Autodesk Fusion 360 part; units mm, degrees
sketch "Sketch1" plane through (0, 0, 0) normal (0, 0, 1) x (1, 0, 0)
  line L0 (4, 2) -> (-4, 2)
  line L1 (-4, 2) -> (-4, -2)
  line L2 (-4, -2) -> (4, -2)
  line L3 (4, -2) -> (4, 2)
  line L4 (4, 2) -> (-4, -2) construction
  line L5 (-4, 2) -> (4, -2) construction
  line L6 (-4, -2) -> (-17, -2)
  line L7 (-17, -2) -> (-17, 10)
  line L8 (-17, 10) -> (0, 10)
  line L9 (-4, 0) -> (-15, 0)
  line L10 (-15, 0) -> (-15, 8)
  line L11 (-15, 8) -> (0, 8)
  line L12 (0, 1.75) -> (0, 22.5)
  line L13 (15, 8) -> (0, 8)
  line L14 (17, 10) -> (0, 10)
  line L15 (17, -2) -> (17, 10)
  line L16 (15, 0) -> (15, 8)
  line L17 (4, 0) -> (15, 0)
  line L18 (4, -2) -> (17, -2)
  line L19 (-17, 10) -> (-23, 10)
  line L20 (-23, 10) -> (-23, 4)
  line L21 (-17, -2) -> (-17, 10)
  circle A0 centre (-20, 7) radius 1.75
  line L22 (-23, 4) -> (-17, -2)
  line L23 (17, 10) -> (23, 10)
  line L24 (23, 10) -> (23, 4)
  line L25 (23, 4) -> (17, -2)
  circle A1 centre (20, 7) radius 1.75
  dimension "d1" = 8
  dimension "d2" = 4
  dimension "d9" = 3.5
extrude "Extrude1" add sketch "Sketch1" along normal blind 2
extrude "Extrude2" add sketch "Sketch1" along normal blind 20 contours L3 L12 L13 L14 L15 L16 L17 L18 | L1 L6 L7 L8 L9 L10 L11 L12 L21
chamfer "Chamfer1" distance 0.8 angle 45 2 edges at (-21.6316, 7.6328, 2) (18.3684, 7.6328, 2)
fillet "Fillet2" radius 4.5 2 edges at (-4, -1, 20) (4, -1, 20)
fillet "Fillet3" radius 2.5 4 edges at (-15, 0, 11) (-15, 8, 11) (15, 8, 11) (15, 0, 11)
Check sheet for the modelled part. Datum: model origin and axes. Units: mm. A direction names the side the tool comes from. Round coordinates to 2 decimals unless told otherwise and drop trailing zeros. Order: outer loops, then holes, each group sorted by start corner. A loop starts at its lowest first (then second) coordinate and runs counter-clockwise, first axis right, second up. Notation, with made-up numbers: (56, 8) - (100, 8) arc R23 cw to (100, 47) - close; hole circle Ø5 at (24.25, 59.5). An arc over 180 degrees is marked (long way). Write item = value, one per line.
Q1. Section check D-D (x = 8). Record the boundary of the cut face in (y, z), and give its area (3 significant figures).
Computed:
outline = (-2, 0) - (10, 0) - (10, 20) - (8, 20) - (8, 2) - (0, 2) - (0, 19.97) - (-2, 19.97) - close
area = 95.9 mm^2
Q2. Thickness scan on line 1 along Y through (x, z) = (-12, 6); line 2 along Z through (x, y) = (1.5, 4); line 3 along X through (y, z) = (8.75, 14.5). Record the ranges inside material, lowest first.
Computed:
line_1 = -2 to 0, 8 to 10
line_2 = 0 to 2
line_3 = -17 to 17
Q3. Go/stop test with flat-tipped pins: pin 1 (1 mm diameter, centred on y = 2.5, z = 14, fed in from -X); pin 2 (2 mm diameter, centred on x = -20, y = 7, fed in from -Z); pin 3 (4 mm diameter, centred on x = 8.5, y = 3.5, fed in from +Z); pin 4 (0.9 mm diameter, centred on y = 3.5, z = 8.5, fed in from +X). Record where each tip stops, or that it passes through.
Computed:
pin_1 = -17
pin_2 = through
pin_3 = 2
pin_4 = 17
Q4. Section check A-A (x = -20). Record the boundary of the cut face in (y, z).
Computed:
outline = (1, 0) - (5.25, 0) - (5.25, 1.2) - (4.45, 2) - (1, 2) - close; (8.75, 0) - (10, 0) - (10, 2) - (9.55, 2) - (8.75, 1.2) - close
Q5. Draft check along Y on faces 4 (the face through (14.287, 7.248, 11.126)), 5 (the face through (0, 10, 10)), 6 (the face through (-23, 7, 1)). Enter one of: pulls with the +Y half, pulls with the -Y half, needs draft (parallel to the pull), parting line crosses it, or undercut.
Computed:
face_4 = undercut
face_5 = pulls with the +Y half
face_6 = needs draft
Q6. Tool access check on faces 1 (the face through (-14.287, 0.752, 11.126)), 2 (the face through (-19, 4, 2)), 3 (the face through (4, -1, 9)). Record the directions out of +Z, -Z, +X, -X, +Y, -Y that give a thin tool (end or side, any length) a straight path to the whole face; none if there is none.
Computed:
face_1 = +Z
face_2 = +Z, -X, +Y, -Y
face_3 = +Z, -Y
Q7. Section check B-B (y = 7). Record the boundary of the cut face in (x, z).
Computed:
outline = (-23, 0) - (-21.75, 0) - (-21.75, 1.2) - (-22.55, 2) - (-23, 2) - close; (-18.25, 0) - (18.25, 0) - (18.25, 1.2) - (17.45, 2) - (17, 2) - (17, 20) - (14.5, 20) - (14.5, 2) - (-14.5, 2) - (-14.5, 20) - (-17, 20) - (-17, 2) - (-17.45, 2) - (-18.25, 1.2) - close; (21.75, 0) - (23, 0) - (23, 2) - (22.55, 2) - (21.75, 1.2) - close
Q8. Section check C-C (z = 11). Record the boundary of the cut face in (x, y).
Computed:
outline = (-17, -2) - (-4, -2) - (-4, 0) - (-12.5, 0) arc R2.5 cw to (-15, 2.5) - (-15, 5.5) arc R2.5 cw to (-12.5, 8) - (12.5, 8) arc R2.5 cw to (15, 5.5) - (15, 2.5) arc R2.5 cw to (12.5, 0) - (4, 0) - (4, -2) - (17, -2) - (17, 10) - (-17, 10) - close
